Check sheet for the modelled part. Datum: model origin and axes. Units: mm. Coordinates: 2 decimals unless noted, no trailing zeros. Loops run counter-clockwise (first coordinate to the right, second up) from the corner with the lowest first, then second, coordinate; pieces in that order, holes last. Notation, with made-up numbers: M -3.5,20.25 L 32.5,20.25 A14 ccw 32.5,30.25 Z; hole C 37,-35.5 d6. An arc over 180 degrees is marked long. Return JSON: item names as keys, results as strings.
from build123d import *

# Parameters (mm, degrees)
F0_R     = 15
F1_DEPTH = 6
F2_R     = 5.99999
F3_T     = 2.5


# Not quite as in the source:
# - a fillet or chamfer is up to 0.001 mm smaller than in the source, because OpenCascade refuses the exact size
# - a shell that OpenCascade refuses in one call is made with other operations: the cavity is built on its own and cut out


with BuildPart() as f1:
    # F0 (on Top) → F1 (new body)
    with BuildSketch(Plane.XY):
        Circle(F0_R)
    extrude(amount=F1_DEPTH)

    # F2 (radius 6 in the source; OpenCascade refuses exactly that, so slightly less here)
    f2_edges = [f1.edges().sort_by_distance(p)[0] for p in [
        (-15, 0, 6),
    ]]
    fillet(f2_edges, radius=F2_R)

    # F3: shell of thickness 2.5, made by hand


with BuildPart() as f3_core1:
    # F3_t2: copy of F1
    add(f1.part)

    # the walls: a layer under each face that stays
    f3_faces = [f3_core1.faces().sort_by_distance(p)[0] for p in [
        (-15, 0, 5e-06),
        (-13.2426436161, 0, 4.2426436161),
        (0, 0, 6),
    ]]
    thicken(f3_faces, amount=-F3_T, mode=Mode.SUBTRACT)


with BuildPart() as f1_1:
    add(f1.part)

    # what is left inside the walls is the cavity
    f3_cavity = [f3_core1.part.solids().sort_by_distance(p)[0] for p in [
        (0, -4.166667, 0.025),
    ]]
    add(f3_cavity, mode=Mode.SUBTRACT)


solid = f1_1.part
1) Go/stop test with flat-tipped pins: pin 1 Ø1 at (x, z) = (6.5, 1) entering from +Y; pin 2 Ø4 at (x, y) = (-4.5, -1) entering from -Z; pin 3 Ø1.5 at (y, z) = (8, 3.5) entering from -X. Record where each tip stops, or that it passes through.
Answers:
{"pin 1": "y = 13.67", "pin 2": "z = 3.5", "pin 3": "x = -12.09"}
2) Scan lines: line 1 along Y through (x, z) = (0, 0.05); line 2 along Z through (x, y) = (8, 2); line 3 along X through (y, z) = (-11.5, 0.75). Record each from-to range of solid material in increasing order. Write a range as [from, to].
Answers:
{"line 1": "[-15, -12.5], [12.5, 15]", "line 2": "[3.5, 6]", "line 3": "[-9.56, -4.69], [4.69, 9.56]"}
3) Section check D-D on z = 0.55. Record the cut outline in (x, y).
Answers:
{"outline": "C 0,0 d29.95; hole C 0,0 d24.91"}
4) Draft check along X on faces 1 (the face through (0, 0, 6)), 2 (the face through (0, 0, 3.5)). Enter one of: +X half, -X half, draft (parallel to the pull), parting line (faces both ways), or undercut.
Answers:
{"face 1": "draft", "face 2": "undercut"}
5) Section check C-C on z = 2.2. Record the cut outline in (x, y), then the cut area to 3 significant figures.
Answers:
{"outline": "C 0,0 d29.16; hole C 0,0 d23.44", "area": "236 mm²"}
